Source: CAD feature listing. Evaluate the final solid. Frame: model axes, mm. Face numbers are marked on the shaded views. A direction names the side the tool comes from. Round coordinates to 2 decimals unless told otherwise and drop trailing zeros. Order: outer loops, then holes, each group sorted by start corner. A loop starts at its lowest first (then second) coordinate and runs counter-clockwise, first axis right, second up. Notation, with made-up numbers: (77.25, -28.5) -> (109.25, -28.5) arc R16 ccw to (109.25, -23.5) -> close; hole circle Ø9 at (76.5, 46). An arc over 180 degrees is marked (long way). Answer as CSV lines item,"result".
from build123d import *

# Parameters (mm, degrees)
SKETCH1_W           = 57.15
SKETCH1_H           = 107.95
BOSS_EXTRUDE1_DEPTH = 2.54
BOSS_EXTRUDE2_DEPTH = 8.89
SKETCH4_R           = 0.635
CUT_EXTRUDE1_DEPTH  = 10.16
SKETCH5_W           = 49.53
SKETCH5_H           = 50.8
BOSS_EXTRUDE3_DEPTH = 7.62
FILLET1_R           = 2.54


with BuildPart() as part:
    # Sketch1 → Boss-Extrude1 (new body)
    with BuildSketch(Plane(origin=(0, 0, 0), x_dir=(1, 0, 0), z_dir=(0, 1, 0))):
        with Locations((28.575, 53.975)):
            Rectangle(SKETCH1_W, SKETCH1_H)
    extrude(amount=BOSS_EXTRUDE1_DEPTH)

    # Sketch2 → Boss-Extrude2 (add)
    with BuildSketch(Plane(origin=(0, 2.54, 0), x_dir=(1, 0, 0), z_dir=(0, 1, 0))):
        with BuildLine():
            Line((8.255, 40.64), (20.955, 40.64))
            ThreePointArc((20.955, 40.64), (22.225, 39.37), (20.955, 38.1))
            Line((20.955, 38.1), (8.255, 38.1))
            ThreePointArc((8.255, 38.1), (6.985, 39.37), (8.255, 40.64))
        make_face()
        with BuildLine():
            Line((48.895, 40.64), (36.195, 40.64))
            ThreePointArc((36.195, 40.64), (34.925, 39.37), (36.195, 38.1))
            Line((36.195, 38.1), (48.895, 38.1))
            ThreePointArc((48.895, 38.1), (50.165, 39.37), (48.895, 40.64))
        make_face()
        with BuildLine():
            Line((8.255, 48.26), (20.955, 48.26))
            ThreePointArc((20.955, 48.26), (22.225, 46.99), (20.955, 45.72))
            Line((20.955, 45.72), (8.255, 45.72))
            ThreePointArc((8.255, 45.72), (6.985, 46.99), (8.255, 48.26))
        make_face()
        with BuildLine():
            Line((48.895, 48.26), (36.195, 48.26))
            ThreePointArc((36.195, 48.26), (34.925, 46.99), (36.195, 45.72))
            Line((36.195, 45.72), (48.895, 45.72))
            ThreePointArc((48.895, 45.72), (50.165, 46.99), (48.895, 48.26))
        make_face()
    extrude(amount=BOSS_EXTRUDE2_DEPTH)

    # Sketch4 → Cut-Extrude1 (cut)
    with BuildSketch(Plane.ZY):
        with Locations((-104.14, 1.27)):
            Circle(SKETCH4_R)
        with Locations(Location((-3.81, 1.27, 0), (0, 0, 180))):
            Circle(SKETCH4_R)
    cut_extrude1 = extrude(amount=-CUT_EXTRUDE1_DEPTH, mode=Mode.SUBTRACT)

    # Mirror1: Cut-Extrude1 across plane
    add(cut_extrude1.mirror(Plane.ZY.offset(-28.575)), mode=Mode.SUBTRACT)

    # Sketch5 → Boss-Extrude3 (add)
    with BuildSketch(Plane(origin=(0, 2.54, 0), x_dir=(1, 0, 0), z_dir=(0, 1, 0))):
        with Locations((28.575, 78.74)):
            Rectangle(SKETCH5_W, SKETCH5_H)
    extrude(amount=BOSS_EXTRUDE3_DEPTH)

    # Fillet1
    fillet1_edges = [part.edges().sort_by_distance(p)[0] for p in [
        (53.34, 6.35, -53.34),
        (53.34, 6.35, -104.14),
        (3.81, 6.35, -104.14),
        (3.81, 6.35, -53.34),
    ]]
    fillet(fillet1_edges, radius=FILLET1_R)


solid = part.part
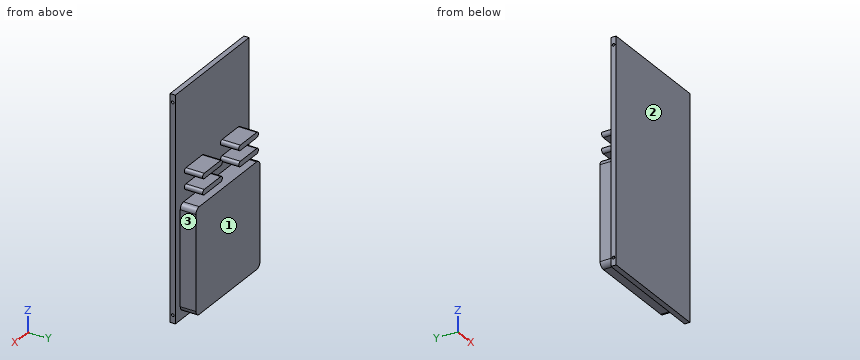
1. Line query: L1, parallel to Z at x = 15, y = 6; L2, parallel to Y at x = 51.25, z = -3.81 (3 decimals); L3, parallel to Z at x = 12, y = 11.25. Output: solid intervals per line, ascending. Write a range as [from, to].
Results below:
L1,"[-104.14, -53.34], [-48.26, -45.72], [-40.64, -38.1]"
L2,"[0, 0.635], [1.905, 2.54]"
L3,"[-48.26, -45.72], [-40.64, -38.1]"
2. Section query C-C on z = -46.99. Return loops of the section in (x, y) (3 decimals).
Results below:
outline,"(0, 0) -> (57.15, 0) -> (57.15, 2.54) -> (50.165, 2.54) -> (50.165, 11.43) -> (34.925, 11.43) -> (34.925, 2.54) -> (22.225, 2.54) -> (22.225, 11.43) -> (6.985, 11.43) -> (6.985, 2.54) -> (0, 2.54) -> close"
3. Pin query (flat end, axial travel): pin 1 (0.6 mm diameter, centred on y = 1.5, z = -104, fed in from -X); pin 2 (6 mm diameter, centred on y = 7, z = -65.5, fed in from +X); pin 3 (3 mm diameter, centred on x = 34, y = 4.5, fed in from -Z). Return the tip coordinate at first contact, or that it passes through.
Results below:
pin 1,"x = 10.16"
pin 2,"x = 53.34"
pin 3,"z = -104.14"
4. Section query D-D on x = 33. Return loops of the section in (y, z).
Results below:
outline,"(0, -107.95) -> (2.54, -107.95) -> (2.54, -104.14) -> (10.16, -104.14) -> (10.16, -53.34) -> (2.54, -53.34) -> (2.54, 0) -> (0, 0) -> close"
5. Reachability of the marked faces 1, 2 and 3 from +Z, -Z, +X, -X, +Y, -Y: full face, straight path, thin tool, end or side. Return the list, or none.
Results below:
face 1,"-Z, +X, -X, +Y"
face 2,"+Z, -Z, +X, -X, -Y"
face 3,"+Z, -Z, +X, +Y"
6. Section query B-B on x = 42. Return loops of the section in (y, z).
Results below:
outline,"(0, -107.95) -> (2.54, -107.95) -> (2.54, -104.14) -> (10.16, -104.14) -> (10.16, -53.34) -> (2.54, -53.34) -> (2.54, -48.26) -> (11.43, -48.26) -> (11.43, -45.72) -> (2.54, -45.72) -> (2.54, -40.64) -> (11.43, -40.64) -> (11.43, -38.1) -> (2.54, -38.1) -> (2.54, 0) -> (0, 0) -> close"
7. Section query A-A on y = 8. Return loops of the section in (x, z) (3 decimals).
Results below:
outline,"(3.81, -101.6) arc R2.54 ccw to (6.35, -104.14) -> (50.8, -104.14) arc R2.54 ccw to (53.34, -101.6) -> (53.34, -55.88) arc R2.54 ccw to (50.8, -53.34) -> (6.35, -53.34) arc R2.54 ccw to (3.81, -55.88) -> close; (8.255, -48.26) -> (20.955, -48.26) arc R1.27 ccw to (20.955, -45.72) -> (8.255, -45.72) arc R1.27 ccw to start; (8.255, -40.64) -> (20.955, -40.64) arc R1.27 ccw to (20.955, -38.1) -> (8.255, -38.1) arc R1.27 ccw to start; (36.195, -48.26) -> (48.895, -48.26) arc R1.27 ccw to (48.895, -45.72) -> (36.195, -45.72) arc R1.27 ccw to start; (36.195, -40.64) -> (48.895, -40.64) arc R1.27 ccw to (48.895, -38.1) -> (36.195, -38.1) arc R1.27 ccw to start"
